The drawing under review shows one solid part. Ordinate dimensions are in mm from its lowest x, y, z. Coordinates: 2 decimals unless noted, no trailing zeros. Write each loop counter-clockwise with the first axis right and the second up, starting at its lowest first coordinate (ties: lowest second). Pieces come first, ordered by that corner, then holes.
1) Add section C-C, the plane y = 1.25. State the section outline as (x, z) points.
2) Add section A-A, the plane z = 32.5. State the section outline as (x, y) points.
3) Add section D-D, the plane z = 58.5. State the section outline as (x, y) points.
4) Add section B-B, the plane x = 32.5. State the section outline as (y, z) points, then the cut area to 3 significant figures.
5) For P1, Ø6, axis at x = 44.5, y = 10.5, coming from the -Z side; P2, Ø1.5, axis at x = 44, y = 2.5, coming from the -Z side; P3, Ø4, axis at x = 29, y = 8.5, coming from the +Z side, all flat-tipped, find the tip position at first contact; note any pin that passes through.
6) Mouldability with a two-part tool opening along Z and no side actions: class the marked faces 1, 2, 3 and 4 as released by +Z, released by -Z, zero draft, split by the parting line, or undercut.
7) For line 1 (Z direction, x = 32.5, y = 5.25); line 2 (Z direction, x = 21.5, y = 7); line 3 (X direction, y = 9.75, z = 58), list the stretches that pass through material, from the lowest coordinate up.
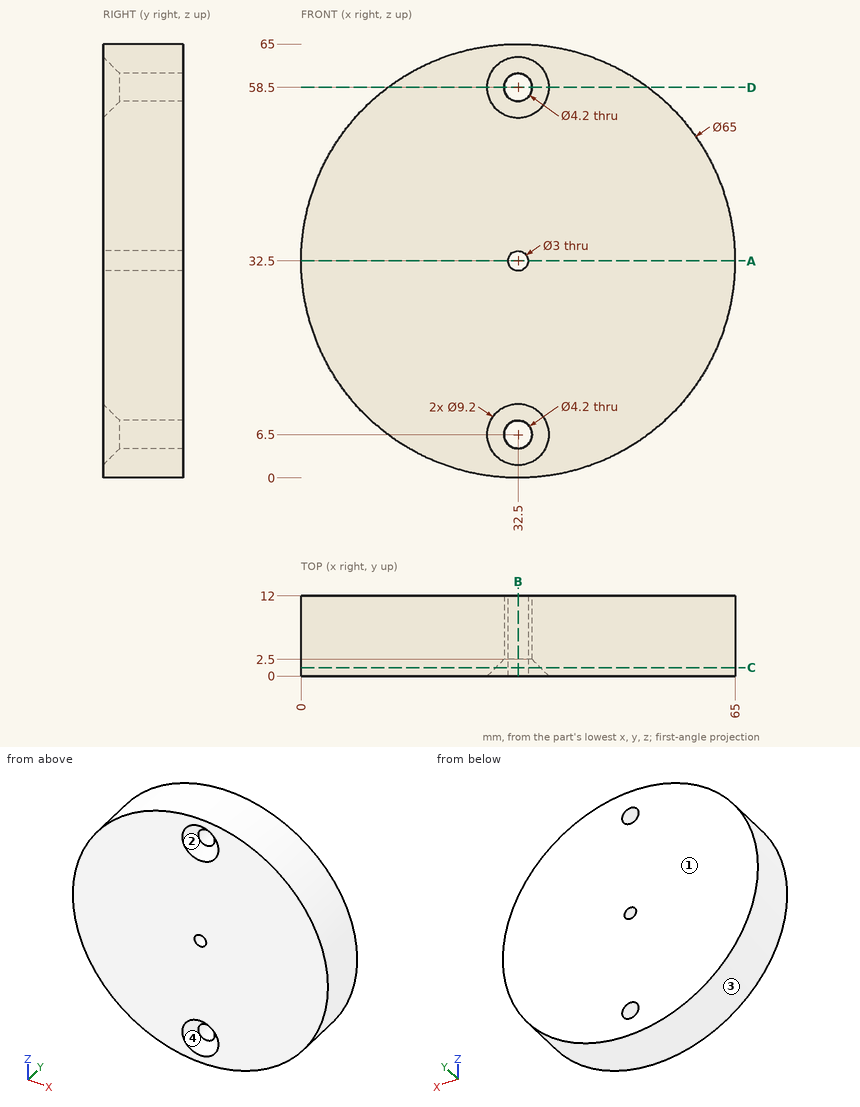
Geometry results:
1. outline: circle Ø65 at (32.5, 32.5); hole circle Ø6.7 at (32.5, 6.5); hole circle Ø6.7 at (32.5, 58.5); hole circle Ø3 at (32.5, 32.5)
2. outline: (0, 0) - (31, 0) - (31, 12) - (0, 12) - close; (34, 0) - (65, 0) - (65, 12) - (34, 12) - close
3. outline: (13, 0) - (27.9, 0) - (30.4, 2.5) - (30.4, 12) - (13, 12) - close; (34.6, 2.5) - (37.1, 0) - (52, 0) - (52, 12) - (34.6, 12) - close
4. outline: (0, 0) - (12, 0) - (12, 4.4) - (2.5, 4.4) - (0, 1.9) - close; (0, 11.1) - (2.5, 8.6) - (12, 8.6) - (12, 31) - (0, 31) - close; (0, 34) - (12, 34) - (12, 56.4) - (2.5, 56.4) - (0, 53.9) - close; (0, 63.1) - (2.5, 60.6) - (12, 60.6) - (12, 65) - (0, 65) - close
4. area: 631 mm2
5. P1: stops at z = 1.27
5. P2: stops at z = 1.83
5. P3: stops at z = 64.97
6. face 1: zero draft
6. face 2: undercut
6. face 3: split by the parting line
6. face 4: undercut
7. line 1: z = 0 to 4.4, 8.6 to 31, 34 to 56.4, 60.6 to 65
7. line 2: z = 1.92 to 63.08
7. line 3: x = 12.35 to 30.46, 34.54 to 52.65
